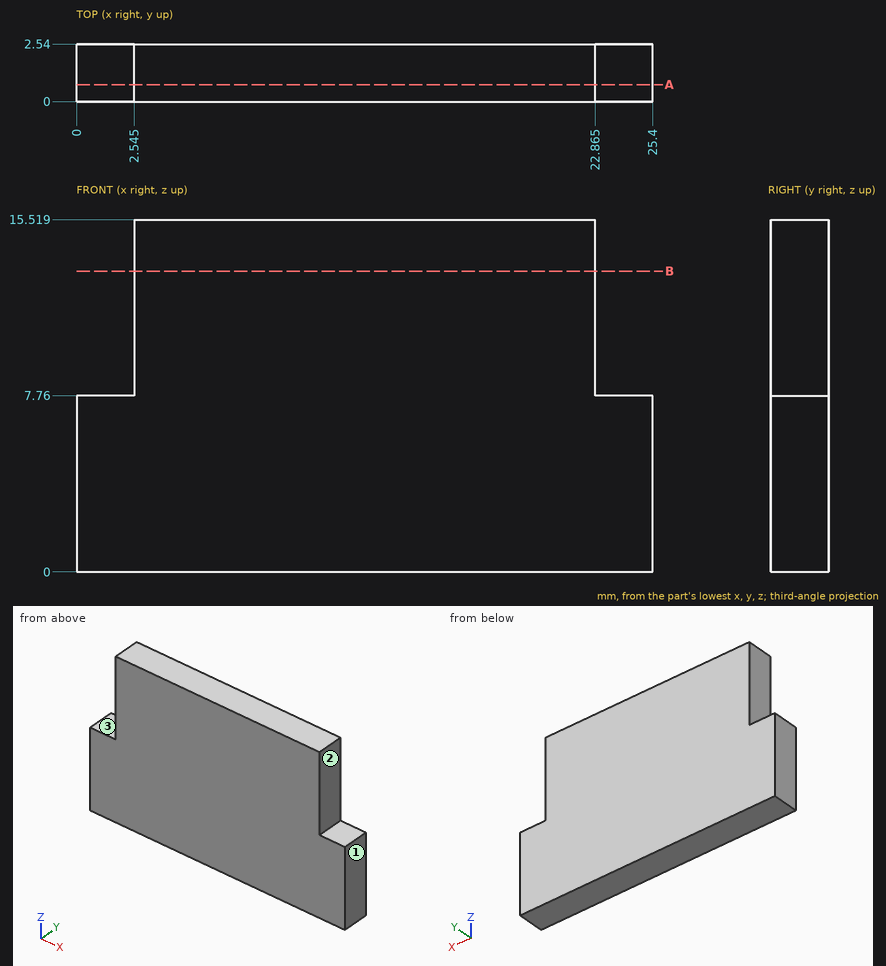
Could you check a few things on this drawing? It's one solid part, dimensions in mm from its lowest x, y, z. A direction names the side the tool comes from. Give positions to 0.01 mm unless a question says otherwise; leave off trailing zeros. Order: outer loops, then holes, each group sorted by start corner. A loop starts at its lowest first (then second) coordinate and runs counter-clockwise, first axis right, second up.
1. Suppose I cut it at A-A (y = 0.75). Write out the boundary of the cut face in (x, z) (1 decimal).
Answers below:
outline: (0, 0) - (25.4, 0) - (25.4, 7.8) - (22.9, 7.8) - (22.9, 15.5) - (2.5, 15.5) - (2.5, 7.8) - (0, 7.8) - close
2. For pin 1 (1.3 mm diameter, centred on x = 1.5, y = 1, fed in from +Z), with a flat end and sliding along its axis, tell me the tip position at first contact or that it passes through.
Answers below:
pin 1: stops at z = 7.76
3. I need wall thicknesses on L1, parallel to Z at x = 1, y = 1.5; L2, parallel to X at y = 0.2, z = 13.5 (1 decimal). Which ranges of each line are inside material? Lowest first, please.
Answers below:
L1: z = 0 to 7.76
L2: x = 2.5 to 22.9
4. Which directions (+Z, -Z, +X, -X, +Y, -Y) give clear straight access to the entire face, cutting with the end or side of a thin tool? Please do the marked faces 1, 2 and 3.
Answers below:
face 1: +Z, -Z, +X, +Y, -Y
face 2: +Z, +X, +Y, -Y
face 3: +Z, -X, +Y, -Y
5. Suppose I cut it at B-B (z = 13.25). Write out the boundary of the cut face in (x, y) (1 decimal).
Answers below:
outline: (2.5, 0) - (22.9, 0) - (22.9, 2.5) - (2.5, 2.5) - close
